The model under review builds one solid part; all positions refer to its coordinate system, in mm. Face numbers are marked on the shaded views. A direction names the side the tool comes from. Round coordinates to 2 decimals unless told otherwise and drop trailing zeros. Order: outer loops, then holes, each group sorted by start corner. A loop starts at its lowest first (then second) coordinate and runs counter-clockwise, first axis right, second up. Notation, with made-up numbers: (6, -17) -> (11, -17) arc R34 ccw to (11, 19) -> close; hole circle Ø4 at (4.25, -8). An arc over 180 degrees is marked (long way). Use a Markdown table: item, result. Add a question column.
```python
from build123d import *

# Parameters (mm, degrees)
SKETCH2_R          = 1.5
CUT_EXTRUDE1_DEPTH = 16.502338533


with BuildPart() as part:
    # Sketch1 → Revolve1 (revolve)
    with BuildSketch(Plane.XY, mode=Mode.PRIVATE) as revolve1_sk:
        Polygon((-2.5, 9.55), (-2.5, 0), (-10, 0), (-10, 3.2), (-4, 3.2), (-4, 9.55), align=None)
    revolve(revolve1_sk.sketch.rotate(Axis((0, 12.509773994, 0), (0, -1, 0)), 270), axis=Axis((0, 12.509773994, 0), (0, -1, 0)))

    # Sketch2 → Cut-Extrude1 (cut, through all)
    with BuildSketch(Plane(origin=(0, 3.2, 0), x_dir=(1, 0, 0), z_dir=(0, 1, 0))):
        with Locations(Location((0, 6, 0), (0, 0, 270))):
            Circle(SKETCH2_R)
        with Locations(Location((5.196152423, -3, 0), (0, 0, 270))):
            Circle(SKETCH2_R)
        with Locations(Location((-5.196152423, -3, 0), (0, 0, 270))):
            Circle(SKETCH2_R)
    extrude(amount=-CUT_EXTRUDE1_DEPTH, mode=Mode.SUBTRACT)


solid = part.part
```
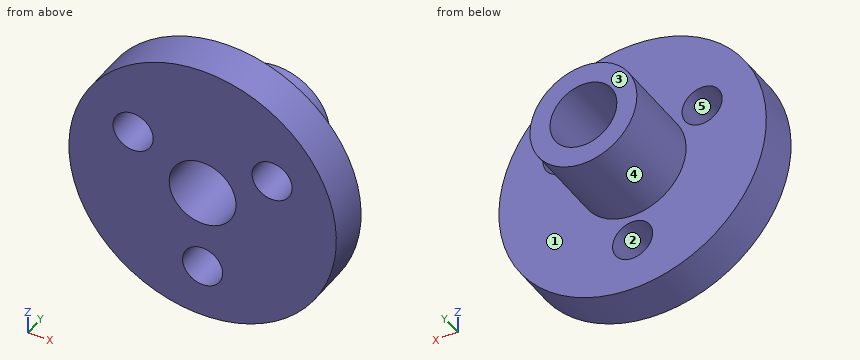
Q1. For pin 1 (4 mm diameter, centred on x = 7, y = 5.5, fed in from -Z); pin 2 (5 mm diameter, centred on y = 2.5, z = 5, fed in from -X); pin 3 (3.5 mm diameter, centred on x = -5.2, z = 3, fed in from +Y), all flat-tipped, find the tip position at first contact; note any pin that passes through.
Q2. Add section D-D, the plane x = -6.25. Give the boundary of the cut face in (y, z), then the cut area to 3 significant figures.
Q3. Add section C-C, the plane z = 3. Give the boundary of the cut face in (x, y), then the cut area to 3 significant figures.
Q4. To check wall thickness, follow line 1 along Z through (x, y) = (-0.5, 2.5); line 2 along X through (y, z) = (4, 0); line 3 along X through (y, z) = (0.9, 3). State the ranges of each line that lie inside material, in increasing order.
Q5. Draft analysis for pull direction X (two halves, no side actions). For the marked faces 3, 4 and 5, state which applies: released by +X, released by -X, zero draft, split by the parting line, or undercut.
Q6. For the marked faces 1 and 2, list the 3-axis set-ups (+Z, -Z, +X, -X, +Y, -Y) from which the entire face can be reached by the end or side of a thin tool; tool diameter is ignored.
Q7. Add section A-A, the plane z = -6. Give the boundary of the cut face in (x, y), then the cut area to 3 significant figures.
Q8. Add section B-B, the plane x = 0. Give the boundary of the cut face in (y, z).
Return value:
| question | item | result |
|---|---|---|
| 1 | pin 1 | through |
| 1 | pin 2 | x = -9.68 |
| 1 | pin 3 | y = 3.2 |
| 2 | outline | (0, -7.81) -> (3.2, -7.81) -> (3.2, 1.93) -> (0, 1.93) -> close; (0, 4.07) -> (3.2, 4.07) -> (3.2, 7.81) -> (0, 7.81) -> close |
| 2 | area | 43.1 mm² |
| 3 | outline | (-9.54, 0) -> (-6.7, 0) -> (-6.7, 3.2) -> (-9.54, 3.2) -> close; (-3.7, 0) -> (3.7, 0) -> (3.7, 3.2) -> (2.65, 3.2) -> (2.65, 9.55) -> (-2.65, 9.55) -> (-2.65, 3.2) -> (-3.7, 3.2) -> close; (6.7, 0) -> (9.54, 0) -> (9.54, 3.2) -> (6.7, 3.2) -> close |
| 3 | area | 75.5 mm² |
| 4 | line 1 | -9.99 to -7.41, -4.59 to -2.45, 2.45 to 9.99 |
| 4 | line 2 | -4 to -2.5, 2.5 to 4 |
| 4 | line 3 | -9.54 to -6.7, -3.7 to 3.7, 6.7 to 9.54 |
| 5 | face 3 | zero draft |
| 5 | face 4 | split by the parting line |
| 5 | face 5 | undercut |
| 6 | face 1 | +Y |
| 6 | face 2 | +Y, -Y |
| 7 | outline | (-8, 0) -> (-1.5, 0) -> (-1.5, 3.2) -> (-8, 3.2) -> close; (1.5, 0) -> (8, 0) -> (8, 3.2) -> (1.5, 3.2) -> close |
| 7 | area | 41.6 mm² |
| 8 | outline | (0, -10) -> (3.2, -10) -> (3.2, -7.5) -> (0, -7.5) -> close; (0, -4.5) -> (3.2, -4.5) -> (3.2, -4) -> (9.55, -4) -> (9.55, -2.5) -> (0, -2.5) -> close; (0, 2.5) -> (9.55, 2.5) -> (9.55, 4) -> (3.2, 4) -> (3.2, 10) -> (0, 10) -> close |
